```python
from build123d import *

# Parameters (mm, degrees)
SKETCH1_R           = 2.667
BOSS_EXTRUDE1_DEPTH = 5.08
SKETCH2_W           = 19.05
SKETCH2_H           = 12.7
BOSS_EXTRUDE2_DEPTH = 0.508
SKETCH4_R           = 1.5875
CUT_EXTRUDE1_DEPTH  = 26.762537724


with BuildPart() as part:
    # Sketch1 → Boss-Extrude1 (new body)
    with BuildSketch(Plane.XY):
        with BuildLine():
            Line((-3.175, 0), (-3.175, 19.05))
            Line((-3.175, 19.05), (-2.54, 19.05))
            Line((-2.54, 19.05), (-2.54, 1.905))
            ThreePointArc((-2.54, 1.905), (0, 3.175), (2.54, 1.905))
            Line((2.54, 1.905), (2.54, 19.05))
            Line((2.54, 19.05), (3.175, 19.05))
            Line((3.175, 19.05), (3.175, 0))
            ThreePointArc((3.175, 0), (0, -3.175), (-3.175, 0))
        make_face()
        Circle(SKETCH1_R, mode=Mode.SUBTRACT)
    extrude(amount=BOSS_EXTRUDE1_DEPTH)

    # Sketch2 → Boss-Extrude2 (add)
    with BuildSketch(Plane(origin=(0, 19.05, 0), x_dir=(1, 0, 0), z_dir=(0, 1, 0))):
        with Locations((0, -2.54)):
            Rectangle(SKETCH2_W, SKETCH2_H)
    extrude(amount=BOSS_EXTRUDE2_DEPTH)

    # Sketch4 → Cut-Extrude1 (cut, through all)
    with BuildSketch(Plane.XZ.offset(-19.05)):
        with Locations(Location((-6.35, 6.35, 0), (0, 0, 270))):
            Circle(SKETCH4_R)
        with Locations(Location((6.35, 6.35, 0), (0, 0, 270))):
            Circle(SKETCH4_R)
        with Locations(Location((6.35, -1.27, 0), (0, 0, 90))):
            Circle(SKETCH4_R)
        with Locations(Location((-6.35, -1.27, 0), (0, 0, 90))):
            Circle(SKETCH4_R)
    extrude(amount=-CUT_EXTRUDE1_DEPTH, mode=Mode.SUBTRACT)


solid = part.part
```
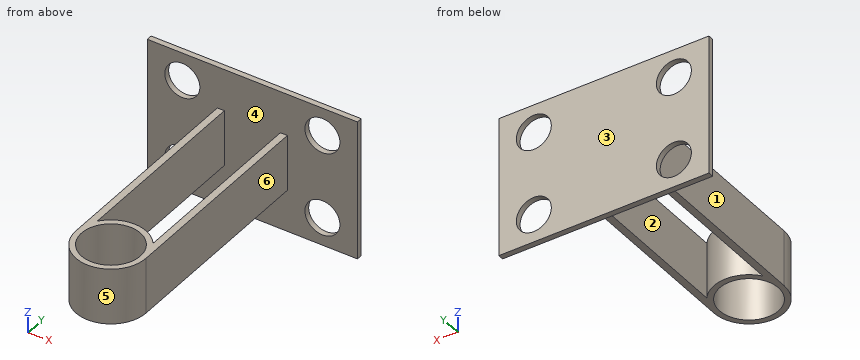
Geometry: final body of the model. Coordinates: model frame, mm. Face numbers are marked on the shaded views. A direction names the side the tool comes from. Round coordinates to 2 decimals unless told otherwise and drop trailing zeros. Order: outer loops, then holes, each group sorted by start corner. A loop starts at its lowest first (then second) coordinate and runs counter-clockwise, first axis right, second up. Notation, with made-up numbers: (73, 80.25) - (118, 80.25) arc R18 cw to (118, 113.25) - close; hole circle Ø8 at (65, 84). An arc over 180 degrees is marked (long way). Write item = value, one per line. Start each with the question number.
Q1. Pull-direction query (X, two-part tool) for the marked faces 4, 5 and 6; classes: +X half, -X half, draft (parallel to the pull), parting line (faces both ways), or undercut.
Q2. Pin query (flat end, axial travel): pin 1 (4 mm diameter, centred on y = 8.5, z = 5.5, fed in from +X) (3 decimals); pin 2 (10 mm diameter, centred on x = -6, y = -0.5, fed in from +Z); pin 3 (1.5 mm diameter, centred on y = 14, z = 3, fed in from -X) (3 decimals). Return the tip coordinate at first contact, or that it passes through.
Q3. Cut plane A-A on x = 0. Return the cut outline in (y, z) (3 decimals).
Q4. Ray query, line 1 (X direction, y = 19.2, z = 6.35) (1 decimal); line 2 (Y direction, x = -2, z = 2); line 3 (X direction, y = 6.75, z = 3) (3 decimals). Return the intervals inside material, ascending. Write a range as from..to.
Q5. Cut plane D-D on x = 4. Return the cut outline in (y, z), and give its area (3 significant figures).
Q6. Cut plane B-B on z = 6.35. Give the number of separate pieces and of enclosed holes in the cut face, and give its area (3 significant figures).
Q7. Access query for the marked faces 1, 2 and 3. Directions: +Z, -Z, +X, -X, +Y, -Y. A direction counts if a zero-diameter tool reaches every point of the face in a straight line with its end or side. Return the directions, or none.
Q8. Cut plane C-C on y = 9.75. Return the cut outline in (x, z) (3 decimals), and give its area (3 significant figures).
Outcome:
q1.face_4 = undercut
q1.face_5 = parting line
q1.face_6 = +X half
q2.pin_1 = 3.175
q2.pin_2 = 5.08
q2.pin_3 = -3.175
q3.outline = (-3.175, 0) - (-2.667, 0) - (-2.667, 5.08) - (-3.175, 5.08) - close; (2.667, 0) - (3.175, 0) - (3.175, 5.08) - (2.667, 5.08) - close; (19.05, -3.81) - (19.558, -3.81) - (19.558, 8.89) - (19.05, 8.89) - close
q4.line_1 = -9.5..-7.9, -4.8..4.8, 7.9..9.5
q4.line_2 = -2.47..-1.76, 1.76..2.47, 19.05..19.56
q4.line_3 = -3.175..-2.54, 2.54..3.175
q5.outline = (19.05, -3.81) - (19.56, -3.81) - (19.56, 8.89) - (19.05, 8.89) - close
q5.area = 6.45 mm^2
q6.separate_pieces = 3
q6.enclosed_holes = 0
q6.area = 6.45 mm^2
q7.face_1 = +Z, -Z, -X, -Y
q7.face_2 = +Z, -Z
q7.face_3 = +Z, -Z, +X, -X, +Y
q8.outline = (-3.175, 0) - (-2.54, 0) - (-2.54, 5.08) - (-3.175, 5.08) - close; (2.54, 0) - (3.175, 0) - (3.175, 5.08) - (2.54, 5.08) - close
q8.area = 6.45 mm^2
